```python
from build123d import *

# Parameters (mm, degrees)
SKETCH1_W                      = 40
SKETCH1_H                      = 137.5
BOSS_EXTRUDE1_DEPTH            = 8
CBORE_FOR_M4_SHCS1_D           = 4.5
CBORE_FOR_M4_SHCS1_CBORE_D     = 8
CBORE_FOR_M4_SHCS1_CBORE_DEPTH = 4
CUT_EXTRUDE1_DEPTH             = 112.893922981
FILLET1_R                      = 10
FILLET2_R                      = 3


with BuildPart() as part:
    # Sketch1 → Boss-Extrude1 (new body)
    with BuildSketch(Plane.XY):
        with Locations((10, -38.75)):
            Rectangle(SKETCH1_W, SKETCH1_H)
        with BuildLine():
            Line((20.25, -52.5), (20.25, -97.5))
            ThreePointArc((20.25, -97.5), (15, -102.75), (9.75, -97.5))
            Line((9.75, -97.5), (9.75, -52.5))
            ThreePointArc((9.75, -52.5), (15, -47.25), (20.25, -52.5))
        make_face(mode=Mode.SUBTRACT)
    extrude(amount=-BOSS_EXTRUDE1_DEPTH)

    # CBORE for M4 SHCS1 (through all)
    with Locations(Plane(origin=(0, 0, -8), x_dir=(1, 0, 0), z_dir=(0, 0, -1))):
        with Locations((0, 0), (23.51, -23.51)):
            CounterBoreHole(CBORE_FOR_M4_SHCS1_D / 2, CBORE_FOR_M4_SHCS1_CBORE_D / 2, CBORE_FOR_M4_SHCS1_CBORE_DEPTH)

    # Sketch6 → Cut-Extrude1 (cut, through all)
    with BuildSketch(Plane.XY):
        with BuildLine():
            Line((-10, -107.5), (4.75, -107.5))
            Line((4.75, -107.5), (4.75, -18.892135624))
            Line((4.75, -18.892135624), (-7.071067812, -7.071067812))
            ThreePointArc((-7.071067812, -7.071067812), (-9.238795322, -3.826834332), (-10, -1.8e-08))
            Line((-10, -1.8e-08), (-10, -107.5))
        make_face()
        with BuildLine():
            Line((-10, 30), (-10, -1.8e-08))
            ThreePointArc((-10, -1.8e-08), (-9.238795329, 3.826834315), (-7.071067812, 7.071067812))
            Line((-7.071067812, 7.071067812), (15.857864376, 30))
            Line((15.857864376, 30), (-10, 30))
        make_face()
        Polygon((25.25, 11.107864376), (25.25, -107.5), (30, -107.5), (30, 15.857864376), align=None)
    extrude(amount=-CUT_EXTRUDE1_DEPTH, mode=Mode.SUBTRACT)

    # Fillet1
    fillet1_edges = [part.edges().sort_by_distance(p)[0] for p in [
        (4.75, -18.892135624, -4),
        (4.75, -107.5, -4),
        (15.857864376, 30, -4),
        (25.25, 11.107864376, -4),
        (25.25, -107.5, -4),
    ]]
    fillet(fillet1_edges, radius=FILLET1_R)

    # Fillet2
    fillet2_edges = [part.edges().sort_by_distance(p)[0] for p in [
        (30, 15.857864376, -4),
        (30, 30, -4),
    ]]
    fillet(fillet2_edges, radius=FILLET2_R)


solid = part.part
```
Input: part model. Units: mm. Frame: model coordinates. A direction names the side the tool comes from. Give positions to 0.01 mm unless a question says otherwise; leave off trailing zeros. Order: outer loops, then holes, each group sorted by start corner. A loop starts at its lowest first (then second) coordinate and runs counter-clockwise, first axis right, second up. Notation, with made-up numbers: M 76.25,69 L 109.25,69 A27 cw 109.25,89 Z; hole C 84.5,-24.75 d3. An arc over 180 degrees is marked long. One line per question, with ' | ' between items. Start each with the question number.
1. Section query A-A (x = 0). Return the cut outline in (y, z), and give its area (3 significant figures).
2. Access query for faces 4 (the face through (29.1, 29.14, -4.06)), 5 (the face through (4.75, -61, -4)), 6 (the face through (20.25, -75, -4)), 7 (the face through (14, -23, -8)), 8 (the face through (-0.867, 3.905, -6.028)). Directions: +Z, -Z, +X, -X, +Y, -Y. A direction counts if a zero-diameter tool reaches every point of the face in a straight line with its end or side. Return the directions, or none.
3. Material intervals for probe 1 along X at (y, z) = (-64.5, -0.75); probe 2 along Y at (x, z) = (23.51, -5.4); probe 3 along X at (y, z) = (-24, -5.25), sorted ascending. Write a range as [from, to].
4. First-contact query: pin 1 Ø5 at (x, y) = (0, 0) entering from -Z; pin 2 Ø4 at (y, z) = (-28, -3.5) entering from +X; pin 3 Ø4 at (x, y) = (0, 0) entering from +Z; pin 4 Ø4 at (y, z) = (-77, -2.5) entering from -X. Flat tips, straight axial feed; report the tip coordinate or a pass-through.
5. Section query D-D (x = 17.5). Return the cut outline in (y, z), and give its area (3 significant figures).
6. Section query C-C (z = -6.25). Return the cut outline in (x, y).
7. Section query B-B (y = -55). Return the cut outline in (x, z).
8. Pull-direction query (X, two-part tool) for faces 1 (the face through (14, -23, 0)), 2 (the face through (3.97, -19.16, -4.06)), 3 (the face through (2, 2, -4)); classes: released by +X, released by -X, zero draft, split by the parting line, or undercut.
Here are the results:
1) outline: M -14.14,-8 L -4,-8 L -4,-4 L -2.25,-4 L -2.25,0 L -14.14,0 Z; M 2.25,-4 L 4,-4 L 4,-8 L 14.14,-8 L 14.14,0 L 2.25,0 Z | area: 176 mm²
2) face 4: +Z, -Z, +X, +Y | face 5: +Z, -Z, -X, -Y | face 6: +Z, -Z | face 7: -Z, +X, -X, +Y, -Y | face 8: -Z
3) probe 1: [4.75, 9.75], [20.25, 25.25] | probe 2: [-103.14, 19.51], [27.51, 30] | probe 3: [4.75, 25.25]
4) pin 1: z = -4 | pin 2: x = 25.25 | pin 3: through | pin 4: x = 4.75
5) outline: M -107.24,-8 L -102.12,-8 L -102.12,0 L -107.24,0 Z; M -47.88,-8 L 29.68,-8 L 29.68,0 L -47.88,0 Z | area: 662 mm²
6) outline: M -7.07,-7.07 L 1.82,-15.96 A10 cw 4.75,-23.03 L 4.75,-97.5 A10 ccw 14.75,-107.5 L 15.25,-107.5 A10 ccw 25.25,-97.5 L 25.25,6.97 A10 cw 28.18,14.04 L 29.12,14.98 A3 ccw 30,17.1 L 30,27 A3 ccw 27,30 L 20,30 A10 ccw 12.93,27.07 L -7.07,7.07 A10 ccw Z; hole C 0,0 d8; hole M 9.75,-97.5 A5.25 ccw 20.25,-97.5 L 20.25,-52.5 A5.25 ccw 9.75,-52.5 Z; hole C 23.51,23.51 d8
7) outline: M 4.75,-8 L 9.75,-8 L 9.75,0 L 4.75,0 Z; M 20.25,-8 L 25.25,-8 L 25.25,0 L 20.25,0 Z
8) face 1: zero draft | face 2: released by -X | face 3: undercut
